Model file for the job. Use its own axes, mm. Round coordinates to 2 decimals unless told otherwise and drop trailing zeros. Loops run counter-clockwise (first coordinate to the right, second up) from the corner with the lowest first, then second, coordinate; pieces in that order, holes last. Notation, with made-up numbers: M 70.5,83 L 91.5,83 A24 ccw 91.5,115 Z; hole C 61,88.5 d6. An arc over 180 degrees is marked long. Use a Markdown table: item, result. Add a question column.
Q1. Cut at D-D (z = 1.2). Give the cut face in (x, y) (3 decimals), plus the area to 3 significant figures.
Q2. Cut at C-C (y = -50.5). Give the cut face in (x, z), plus the area to 3 significant figures.
Q3. Cut at A-A (y = 0). Give the cut face in (x, z).
Q4. Cut at B-B (x = 0). Give the cut face in (y, z).
Q5. Probe line 1 (Y direction, x = 0, z = 0.6); line 2 (Y direction, x = -2, z = 0.15); line 3 (Y direction, x = 18.5, z = 1.05). List the from-to ranges inside material, lowest first. Write a range as from..to.
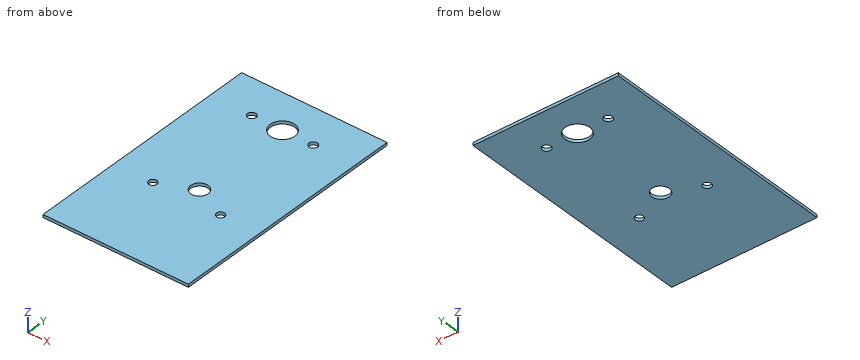
from build123d import *

# Parameters (mm, degrees)
SKETCH1_W           = 75
SKETCH1_H           = 125
SKETCH1_R           = 4.5
SKETCH1_R_2         = 6.35
SKETCH1_R_3         = 2.1
SKETCH1_R_4         = 2.1828125
BOSS_EXTRUDE1_DEPTH = 1.524


with BuildPart() as part:
    # Sketch1 → Boss-Extrude1 (new body)
    with BuildSketch(Plane.XY):
        with Locations((0, -42.5)):
            Rectangle(SKETCH1_W, SKETCH1_H)
        with Locations((0, -52.299124508)):
            Circle(SKETCH1_R, mode=Mode.SUBTRACT)
        Circle(SKETCH1_R_2, mode=Mode.SUBTRACT)
        with Locations((-17.5, -60.299124508)):
            Circle(SKETCH1_R_3, mode=Mode.SUBTRACT)
        with Locations((17.5, -60.299124508)):
            Circle(SKETCH1_R_3, mode=Mode.SUBTRACT)
        with Locations((-15.875, 0)):
            Circle(SKETCH1_R_4, mode=Mode.SUBTRACT)
        with Locations((15.875, 0)):
            Circle(SKETCH1_R_4, mode=Mode.SUBTRACT)
    extrude(amount=BOSS_EXTRUDE1_DEPTH)


solid = part.part
Checked values:
| question | item | result |
|---|---|---|
| 1 | outline | M -37.5,-105 L 37.5,-105 L 37.5,20 L -37.5,20 Z; hole C -17.5,-60.299 d4.2; hole C -15.875,0 d4.366; hole C 0,0 d12.7; hole C 0,-52.299 d9; hole C 15.875,0 d4.366; hole C 17.5,-60.299 d4.2 |
| 1 | area | 9,130 mm^2 |
| 2 | outline | M -37.5,0 L -4.12,0 L -4.12,1.52 L -37.5,1.52 Z; M 4.12,0 L 37.5,0 L 37.5,1.52 L 4.12,1.52 Z |
| 2 | area | 102 mm^2 |
| 3 | outline | M -37.5,0 L -18.06,0 L -18.06,1.52 L -37.5,1.52 Z; M -13.69,0 L -6.35,0 L -6.35,1.52 L -13.69,1.52 Z; M 6.35,0 L 13.69,0 L 13.69,1.52 L 6.35,1.52 Z; M 18.06,0 L 37.5,0 L 37.5,1.52 L 18.06,1.52 Z |
| 4 | outline | M -105,0 L -56.8,0 L -56.8,1.52 L -105,1.52 Z; M -47.8,0 L -6.35,0 L -6.35,1.52 L -47.8,1.52 Z; M 6.35,0 L 20,0 L 20,1.52 L 6.35,1.52 Z |
| 5 | line 1 | y = -105..-56.8, -47.8..-6.35, 6.35..20 |
| 5 | line 2 | y = -105..-56.33, -48.27..-6.03, 6.03..20 |
| 5 | line 3 | y = -105..-62.15, -58.45..20 |
